```python
from build123d import *

# Parameters (mm, degrees)
SKETCH_1_W      = 80
SKETCH_1_H      = 20
SKETCH_1_R      = 3
EXTRUDE_1_DEPTH = 5
SKETCH_2_W      = 40
SKETCH_2_H      = 20
EXTRUDE_2_DEPTH = 20
SKETCH_3_W      = 80
SKETCH_3_H      = 20
SKETCH_3_R      = 5
SKETCH_3_R_2    = 2.5
EXTRUDE_3_DEPTH = 5


with BuildPart() as part:
    # 草图1 → 凸台-拉伸1 (new body)
    with BuildSketch(Plane(origin=(0, 0, 0), x_dir=(1, 0, 0), z_dir=(0, 1, 0))):
        Rectangle(SKETCH_1_W, SKETCH_1_H)
        with Locations(Location((-30, 0, 0), (0, 0, 270))):
            Circle(SKETCH_1_R, mode=Mode.SUBTRACT)
        with Locations(Location((30, 0, 0), (0, 0, 270))):
            Circle(SKETCH_1_R, mode=Mode.SUBTRACT)
    extrude(amount=EXTRUDE_1_DEPTH)

    # 草图2 → 凸台-拉伸2 (add)
    with BuildSketch(Plane(origin=(0, 5, 0), x_dir=(1, 0, 0), z_dir=(0, 1, 0))):
        Rectangle(SKETCH_2_W, SKETCH_2_H)
    extrude(amount=EXTRUDE_2_DEPTH)

    # 草图3 → 凸台-拉伸3 (add)
    with BuildSketch(Plane.XZ):
        Rectangle(SKETCH_3_W, SKETCH_3_H)
        with Locations(Location((-30, 0, 0), (0, 0, 270))):
            Circle(SKETCH_3_R, mode=Mode.SUBTRACT)
        with Locations(Location((30, 0, 0), (0, 0, 270))):
            Circle(SKETCH_3_R, mode=Mode.SUBTRACT)
        with Locations(Location((0, 0, 0), (0, 0, 270))):
            Circle(SKETCH_3_R_2, mode=Mode.SUBTRACT)
    extrude(amount=EXTRUDE_3_DEPTH)


solid = part.part
```
Work out the finished part from the listing and answer in its coordinate system (mm). A direction names the side the tool comes from. Round coordinates to 2 decimals unless told otherwise and drop trailing zeros. Write each loop counter-clockwise with the first axis right and the second up, starting at its lowest first coordinate (ties: lowest second). Pieces come first, ordered by that corner, then holes. Notation, with made-up numbers: (48, -4) - (102, -4) arc R19 ccw to (102, 19) - close; hole circle Ø1 at (15, 21). An arc over 180 degrees is marked (long way). Return JSON: item names as keys, results as strings. Group by question number.
Q1. The part is cut by section B-B on y = 0.75. Write down the section's boundary in (x, z).
Q2. Find the intervals of material crossed by L1, parallel to X at y = -3.8, z = 0; L2, parallel to X at y = 2.6, z = 0; L3, parallel to X at y = 6, z = -3, in increasing order.
Q3. The part is cut by section C-C on z = -1. Write down the section's boundary in (x, y).
Q4. The mould has two halves that part along X. Classify faces 4 (the flat face through (40, 0, 0)), 5 (the flat face through (29.9, 0, 3.3)), 6 (the flat face through (0, 25, 0)): released by +X, released by -X, zero draft, split by the parting line, or undercut.
Q5. The part is cut by section D-D on x = 0. Write down the section's boundary in (y, z), then the cut area to 3 significant figures.
Q6. The part is cut by section A-A on x = -30. Write down the section's boundary in (y, z).
Q7. Each of these flat-tipped pins is pushed along its axis until it touches: pin 1 Ø2 at (y, z) = (10.5, 2.5) entering from +X; pin 2 Ø12 at (y, z) = (19, 0) entering from -X; pin 3 Ø8 at (x, z) = (-30, 0) entering from +Y; pin 4 Ø5 at (x, z) = (30, 0) entering from -Y. Where does it stop, or does it pass through?
Q8. For faces 1 (the cylindrical face through (-34.88, -2.46, 1.08)), 2 (the flat face through (-32.4, 5, -2.4)), 3 (the flat face through (27.6, 5, -2.4)), determine the directions among +Z, -Z, +X, -X, +Y, -Y from which every point of the face is accessible in a straight line to the end or side of a thin tool.
Solved:
{
 "1": {"outline": "(-40, -10) - (40, -10) - (40, 10) - (-40, 10) - close; hole circle Ø6 at (-30, 0); hole circle Ø6 at (30, 0)"},
 "2": {"L1": "-40 to -35, -25 to -2.5, 2.5 to 25, 35 to 40", "L2": "-40 to -33, -27 to 27, 33 to 40", "L3": "-20 to 20"},
 "3": {"outline": "(-40, -5) - (-34.9, -5) - (-34.9, 0) - (-32.83, 0) - (-32.83, 5) - (-40, 5) - close; (-27.17, 0) - (-25.1, 0) - (-25.1, -5) - (-2.29, -5) - (-2.29, 0) - (2.29, 0) - (2.29, -5) - (25.1, -5) - (25.1, 0) - (27.17, 0) - (27.17, 5) - (20, 5) - (20, 25) - (-20, 25) - (-20, 5) - (-27.17, 5) - close; (32.83, 0) - (34.9, 0) - (34.9, -5) - (40, -5) - (40, 5) - (32.83, 5) - close"},
 "4": {"face 4": "released by +X", "face 5": "undercut", "face 6": "zero draft"},
 "5": {"outline": "(-5, -10) - (25, -10) - (25, 10) - (-5, 10) - (-5, 2.5) - (0, 2.5) - (0, -2.5) - (-5, -2.5) - close", "area": "575 mm²"},
 "6": {"outline": "(-5, -10) - (5, -10) - (5, -3) - (0, -3) - (0, -5) - (-5, -5) - close; (-5, 5) - (0, 5) - (0, 3) - (5, 3) - (5, 10) - (-5, 10) - close"},
 "7": {"pin 1": "x = 20", "pin 2": "x = -20", "pin 3": "y = 5", "pin 4": "through"},
 "8": {"face 1": "-Y", "face 2": "+Z, -Z, -X, +Y", "face 3": "+Z, -Z, +X, +Y"}
}
